from build123d import *

# Parameters (mm, degrees)
SKETCH2_W           = 106.2
SKETCH2_H           = 108
BOSS_EXTRUDE1_DEPTH = 38.1
SKETCH3_W           = 25.19
SKETCH3_H           = 108
BOSS_EXTRUDE2_DEPTH = 45.43
SKETCH5_W           = 12.86
SKETCH5_H           = 108
BOSS_EXTRUDE4_DEPTH = 3.2
SKETCH6_W           = 151.63
SKETCH6_H           = 108
CUT_EXTRUDE1_DEPTH  = 21
SKETCH7_W           = 151.63
SKETCH7_H           = 108
BOSS_EXTRUDE5_DEPTH = 59


with BuildPart() as part:
    # Sketch2 → Boss-Extrude1 (new body)
    with BuildSketch(Plane.XY.offset(5.492308275)):
        with Locations((19.206268294, 5.678957245)):
            Rectangle(SKETCH2_W, SKETCH2_H)
    extrude(amount=BOSS_EXTRUDE1_DEPTH)

    # Sketch3 → Boss-Extrude2 (add)
    with BuildSketch(Plane.ZY.offset(33.893731706)):
        with Locations((30.997308275, 5.678957245)):
            Rectangle(SKETCH3_W, SKETCH3_H)
    extrude(amount=BOSS_EXTRUDE2_DEPTH)

    # Sketch5 → Boss-Extrude4 (add)
    with BuildSketch(Plane(origin=(0, 0, 18.402308275), x_dir=(-1, 0, 0), z_dir=(0, 0, -1))):
        with Locations((72.893731706, 5.678957245)):
            Rectangle(SKETCH5_W, SKETCH5_H)
    extrude(amount=BOSS_EXTRUDE4_DEPTH)

    # Sketch6 → Cut-Extrude1 (cut)
    with BuildSketch(Plane.XY.offset(43.592308275)):
        with Locations((-3.508731706, 5.678957245)):
            Rectangle(SKETCH6_W, SKETCH6_H)
    extrude(amount=-CUT_EXTRUDE1_DEPTH, mode=Mode.SUBTRACT)

    # Sketch7 → Boss-Extrude5 (add)
    with BuildSketch(Plane.XY.offset(22.592308275)):
        with Locations((-3.508731706, 5.678957245)):
            Rectangle(SKETCH7_W, SKETCH7_H)
    extrude(amount=BOSS_EXTRUDE5_DEPTH)


solid = part.part
Read the model definition and answer for the solid it produces. Units are mm, in the model's axes. A direction names the side the tool comes from. Give positions to 0.01 mm unless a question says otherwise; leave off trailing zeros. Write each loop counter-clockwise with the first axis right and the second up, starting at its lowest first coordinate (ties: lowest second). Pieces come first, ordered by that corner, then holes. Notation, with made-up numbers: (50, 88.5) - (95, 88.5) arc R28 cw to (95, 121.5) - close; hole circle Ø9 at (9.5, 23.5). An arc over 180 degrees is marked (long way). Answer in a Markdown table with one row per item. Add a question column.
Item 1: Section A-A, the plane y = 19.5 is taken. Write down the section's boundary in (x, z).
Item 2: Determine the mould class of faces 3 (the face through (-66.464, 5, 17)), 4 (the face through (-50, 5, 18.402)), 5 (the face through (-73, 6, 15.202)), 6 (the face through (-79.324, 5, 48)) for opening direction X: pulls with the +X half, pulls with the -X half, needs draft (parallel to the pull), parting line crosses it, or undercut.
Item 3: A tool of negligible diameter and unlimited length cuts with its end or side. For faces 1 (the face through (18, 6, 5.492)), 2 (the face through (-33.894, 5, 12)), from which of +Z, -Z, +X, -X, +Y, -Y can it reach the whole face along a straight path? Write none if from no direction.
Item 4: Find the intervals of material crossed by L1, parallel to X at y = -10, z = 11; L2, parallel to Z at x = -71, y = -35; L3, parallel to X at y = -2, z = 16.5, in increasing order.
Item 5: Flat-ended cylindrical pins translate along their axes: P1, Ø14, axis at x = -70, y = -4.5, coming from the -Z side; P2, Ø4, axis at y = 12, z = 12.5, coming from the -X side. Find the tip coordinate at first contact, or state that the pin passes through.
Item 6: Section B-B, the plane x = -58.5 is taken. Write down the section's boundary in (y, z).
Recorded:
| question | item | result |
|---|---|---|
| 1 | outline | (-79.32, 15.2) - (-66.46, 15.2) - (-66.46, 18.4) - (-33.89, 18.4) - (-33.89, 5.49) - (72.31, 5.49) - (72.31, 81.59) - (-79.32, 81.59) - close |
| 2 | face 3 | undercut |
| 2 | face 4 | undercut |
| 2 | face 5 | needs draft |
| 2 | face 6 | pulls with the -X half |
| 3 | face 1 | -Z, +X, -X, +Y, -Y |
| 3 | face 2 | -Z, +Y, -Y |
| 4 | L1 | x = -33.89 to 72.31 |
| 4 | L2 | z = 15.2 to 81.59 |
| 4 | L3 | x = -79.32 to -66.46, -33.89 to 72.31 |
| 5 | P1 | stops at z = 15.2 |
| 5 | P2 | stops at x = -33.89 |
| 6 | outline | (-48.32, 18.4) - (59.68, 18.4) - (59.68, 81.59) - (-48.32, 81.59) - close |
